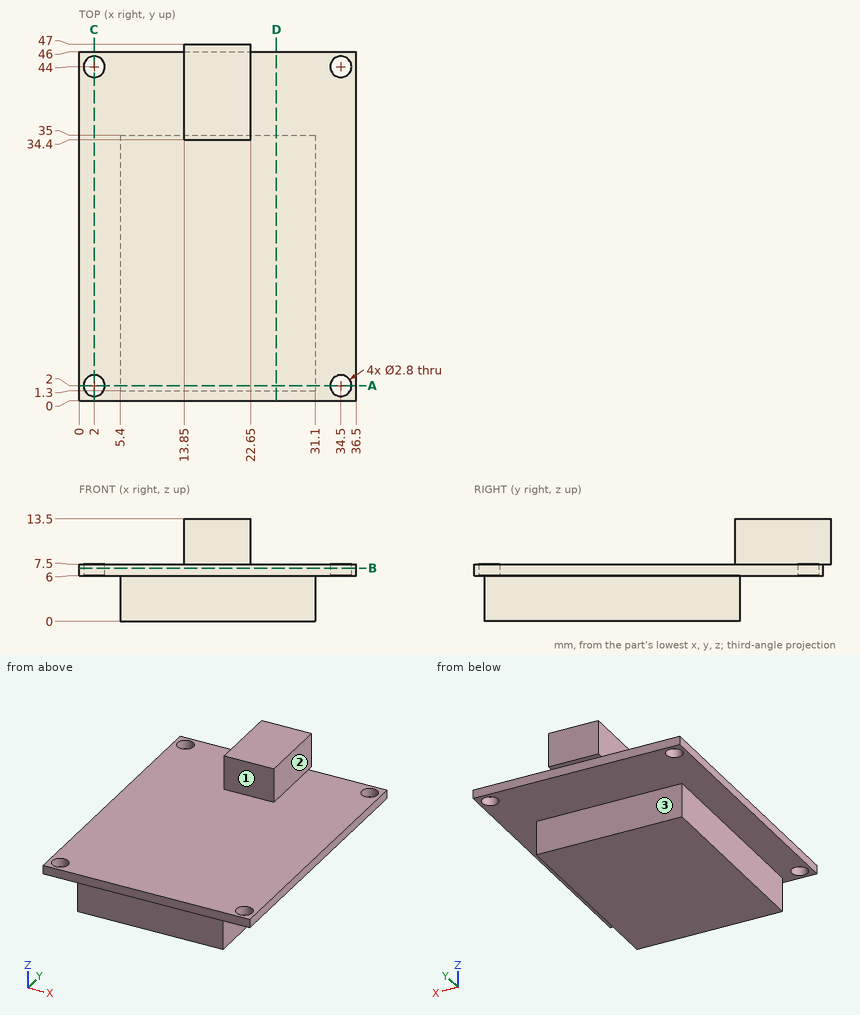
Here's the drawing with two shaded views (mm, measured from the low corner). I have some questions. A direction names the side the tool comes from. Give positions to 0.01 mm unless a question says otherwise; leave off trailing zeros. Loops run counter-clockwise (first coordinate to the right, second up) from the corner with the lowest first, then second, coordinate; pieces in that order, holes last. Notation, with made-up numbers: (84.5, 41.5) - (123.5, 41.5) arc R30 cw to (123.5, 76.5) - close; hole circle Ø3 at (61.5, -12). An arc over 180 degrees is marked (long way). Return JSON: item names as keys, results as strings.
1. If I drill on line 1 (Y direction, x = 2, z = 7); line 2 (Y direction, x = 13.5, z = 1.25); line 3 (X direction, y = 17, z = 0.5), over which ranges is the centre line in solid material (lowest first)?
Output values:
{"line 1": "y = 0 to 0.6, 3.4 to 42.6, 45.4 to 46", "line 2": "y = 1.3 to 35", "line 3": "x = 5.4 to 31.1"}
2. I want a section at C-C on x = 2. Please give me the cut outline in (y, z), and give its area (3 significant figures).
Output values:
{"outline": "(0, 6) - (0.6, 6) - (0.6, 7.5) - (0, 7.5) - close; (3.4, 6) - (42.6, 6) - (42.6, 7.5) - (3.4, 7.5) - close; (45.4, 6) - (46, 6) - (46, 7.5) - (45.4, 7.5) - close", "area": "60.6 mm²"}
3. I want a section at A-A on y = 2. Please give me the cut outline in (x, z).
Output values:
{"outline": "(0, 6) - (0.6, 6) - (0.6, 7.5) - (0, 7.5) - close; (3.4, 6) - (5.4, 6) - (5.4, 0) - (31.1, 0) - (31.1, 6) - (33.1, 6) - (33.1, 7.5) - (3.4, 7.5) - close; (35.9, 6) - (36.5, 6) - (36.5, 7.5) - (35.9, 7.5) - close"}
4. I'm going to push flat-ended pins straight in: pin 1 Ø0.5 at (x, y) = (16.5, 46.5) entering from -Z; pin 2 Ø1 at (x, z) = (19.5, 2) entering from -Y; pin 3 Ø1.8 at (y, z) = (25, 1.5) entering from +X. Where does each tip first touch, or does it pass through?
Output values:
{"pin 1": "stops at z = 7.5", "pin 2": "stops at y = 1.3", "pin 3": "stops at x = 31.1"}
5. I want a section at B-B on z = 7. Please give me the cut outline in (x, y), and give its area (3 significant figures).
Output values:
{"outline": "(0, 0) - (36.5, 0) - (36.5, 46) - (0, 46) - close; hole circle Ø2.8 at (2, 2); hole circle Ø2.8 at (2, 44); hole circle Ø2.8 at (34.5, 2); hole circle Ø2.8 at (34.5, 44)", "area": "1,650 mm²"}
6. For the marked faces 1, 2 and 3, which set-ups out of +Z, -Z, +X, -X, +Y, -Y let a thin tool reach every point of the face, with its end or its side?
Output values:
{"face 1": "+Z, +X, -X, -Y", "face 2": "+Z, +X, +Y, -Y", "face 3": "-Z, +X, -X, +Y"}
7. I want a section at D-D on x = 26. Please give me the cut outline in (y, z).
Output values:
{"outline": "(0, 6) - (1.3, 6) - (1.3, 0) - (35, 0) - (35, 6) - (46, 6) - (46, 7.5) - (0, 7.5) - close"}
